Answer from the drawing. Dimensions are ordinates in mm from the lowest x, y and z of the part. A direction names the side the tool comes from. Give positions to 0.01 mm unless a question says otherwise; leave off trailing zeros. Write each loop counter-clockwise with the first axis right and the second up, starting at its lowest first coordinate (ties: lowest second). Pieces come first, ordered by that corner, then holes. Notation, with made-up numbers: (-12.75, -21) -> (21.25, -21) arc R23 ccw to (21.25, 17) -> close; hole circle Ø6 at (-9.75, 85.25). An arc over 180 degrees is marked (long way). Put each result on its own line as item: value. Start each with the question number.
1) A cutting plane is placed at C-C (z = 6). Write down the section's boundary in (x, y).
2) Flat-ended cylindrical pins translate along their axes: pin 1 Ø3 at (x, z) = (2, 9) entering from +Y; pin 2 Ø1 at (y, z) = (2, 49) entering from +X. Find the tip coordinate at first contact, or state that the pin passes through.
3) For the marked faces 1 and 2, determine the directions among +Z, -Z, +X, -X, +Y, -Y from which every point of the face is accessible in a straight line to the end or side of a thin tool.
4) Find the intervals of material crossed by line 1 along Z through (x, y) = (6.5, 6); line 2 along X through (y, z) = (4.25, 23); line 3 along Y through (x, z) = (4.5, 6.5), in increasing order. Write a range as from..to.
5) A cutting plane is placed at A-A (x = 4). Write down the section's boundary in (y, z).
6) A cutting plane is placed at D-D (z = 54). Write down the section's boundary in (x, y).
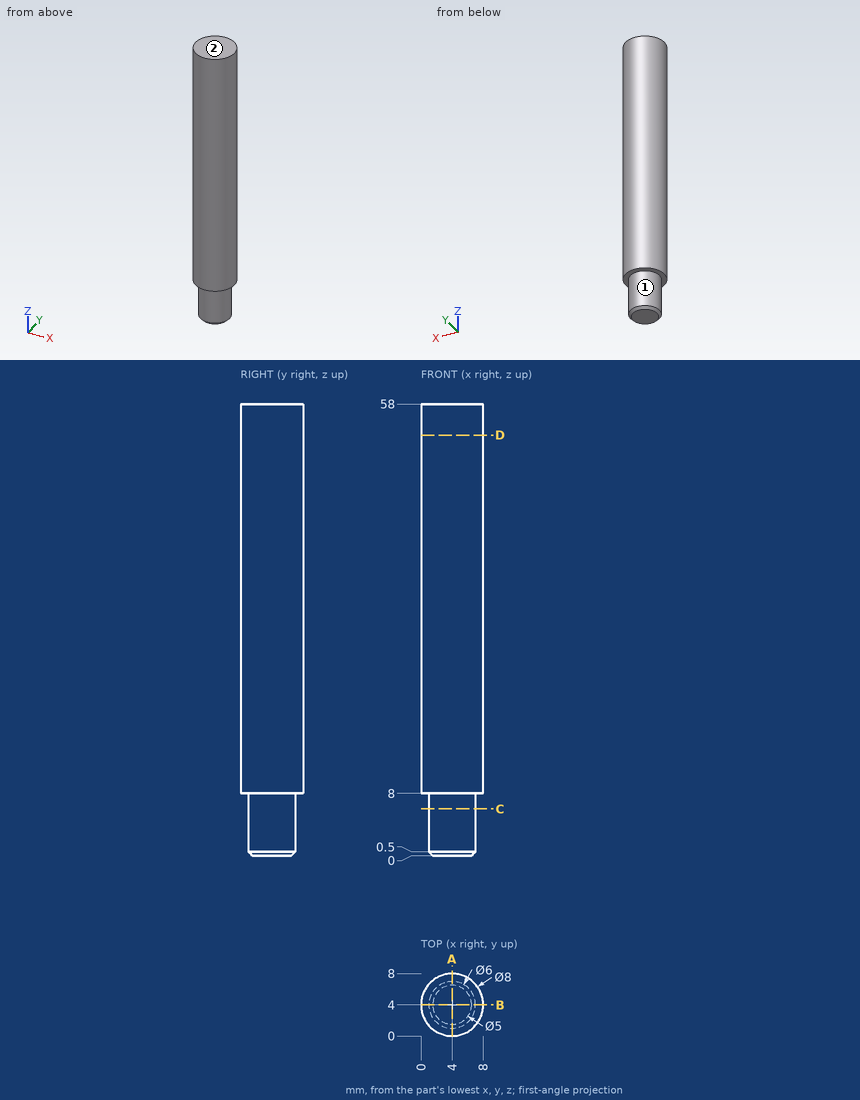
Reply:
1. outline: circle Ø6 at (4, 4)
2. pin 1: stops at y = 7.97
2. pin 2: stops at x = 7.71
3. face 1: -Z
3. face 2: +Z, +X, -X, +Y, -Y
4. line 1: z = 8..58
4. line 2: x = 0.01..7.99
4. line 3: y = 1.04..6.96
5. outline: (0, 8) -> (1, 8) -> (1, 0.5) -> (1.5, 0) -> (6.5, 0) -> (7, 0.5) -> (7, 8) -> (8, 8) -> (8, 58) -> (0, 58) -> close
6. outline: circle Ø8 at (4, 4)
